from build123d import *

# Parameters (mm, degrees)
BOSS_EXTRUDE1_DEPTH      = 21.59
BOSS_EXTRUDE1_DEPTH_BACK = 21.59
SKETCH1_R                = 5.715
SKETCH3_W                = 43.18
SKETCH3_H                = 11.43
BOSS_EXTRUDE3_DEPTH      = 12.7
SKETCH4_W                = 36.83
SKETCH4_H                = 15.24
BOSS_EXTRUDE4_DEPTH      = 24.13
SKETCH7_W                = 36.83
SKETCH7_H                = 12.7
BOSS_EXTRUDE5_DEPTH      = 10.795
SKETCH5_R                = 3.175
CUT_EXTRUDE1_DEPTH       = 52.230767367
CUT_EXTRUDE5_DEPTH       = 52.230767367
FILLET1_R                = 2.54
CUT_EXTRUDE6_DEPTH       = 6.35
CUT_EXTRUDE6_DEPTH_BACK  = 6.35
SKETCH10_W               = 22.86
SKETCH10_H               = 25.4
SKETCH11_R               = 1.778
CUT_EXTRUDE7_DEPTH       = 36.017241825
SKETCH24_W               = 48.26
SKETCH24_H               = 24.13
BOSS_EXTRUDE6_DEPTH      = 2.54
SKETCH17_W               = 12.7
SKETCH17_H               = 3.175
CUT_EXTRUDE9_DEPTH       = 8.89
SKETCH18_W               = 9.525
SKETCH18_H               = 6.927192993
CUT_EXTRUDE13_DEPTH      = 45.508925283
CHAMFER1_SIZE            = 1.27
FILLET2_R                = 1.27


with BuildPart() as part:
    # Sketch1 → Boss-Extrude1 (new, two sides: drawn at the far end of the back side and taken through both)
    with BuildSketch(Plane(origin=(0, 0, 0), x_dir=(0, 0, -1), z_dir=(1, 0, 0)).offset(-BOSS_EXTRUDE1_DEPTH_BACK)):
        Circle(SKETCH1_R)
    extrude(amount=BOSS_EXTRUDE1_DEPTH + BOSS_EXTRUDE1_DEPTH_BACK)

    # Sketch3 → Boss-Extrude3 (add)
    with BuildSketch(Plane(origin=(0, 0, 0), x_dir=(1, 0, 0), z_dir=(0, 1, 0))):
        Rectangle(SKETCH3_W, SKETCH3_H)
    extrude(amount=BOSS_EXTRUDE3_DEPTH)


with BuildPart() as body_2:
    # Sketch4 → Boss-Extrude4 (new body)
    with BuildSketch(Plane.XY):
        with Locations((0, 5.08)):
            Rectangle(SKETCH4_W, SKETCH4_H)
    extrude(amount=BOSS_EXTRUDE4_DEPTH)


with BuildPart() as body_3:
    # Sketch7 → Boss-Extrude5 (new body)
    with BuildSketch(Plane.XZ.offset(2.54)):
        with Locations((0, 17.78)):
            Rectangle(SKETCH7_W, SKETCH7_H)
    extrude(amount=BOSS_EXTRUDE5_DEPTH)


with BuildPart() as cut_extrude1_tool:
    # Sketch5 → Cut-Extrude1 (new, through all)
    with BuildSketch(Plane.ZY.offset(21.59)):
        Circle(SKETCH5_R)
    extrude(amount=-CUT_EXTRUDE1_DEPTH)


with BuildPart() as part_1:
    add(part.part)

    # Cut-Extrude1: cut by cut_extrude1_tool
    add(cut_extrude1_tool.part, mode=Mode.SUBTRACT)


with BuildPart() as body_2_1:
    add(body_2.part)

    # Cut-Extrude1: cut by cut_extrude1_tool
    add(cut_extrude1_tool.part, mode=Mode.SUBTRACT)


with BuildPart() as cut_extrude5_tool:
    # Sketch6 → Cut-Extrude5 (new, through all)
    with BuildSketch(Plane(origin=(21.59, 0, 0), x_dir=(0, 0, -1), z_dir=(1, 0, 0))):
        with BuildLine():
            ThreePointArc((-19.445417037, -14.2875), (-24.13, 0), (-19.445417037, 14.2875))
            Line((-19.445417037, 14.2875), (-27.94, 14.2875))
            Line((-27.94, 14.2875), (-27.94, -14.2875))
            Line((-27.94, -14.2875), (-19.445417037, -14.2875))
        make_face()
    extrude(amount=-CUT_EXTRUDE5_DEPTH)


with BuildPart() as body_2_2:
    add(body_2_1.part)

    # Cut-Extrude5: cut by cut_extrude5_tool
    add(cut_extrude5_tool.part, mode=Mode.SUBTRACT)


with BuildPart() as body_3_1:
    add(body_3.part)

    # Cut-Extrude5: cut by cut_extrude5_tool
    add(cut_extrude5_tool.part, mode=Mode.SUBTRACT)

    # Fillet1
    fillet1_edges = [body_3_1.edges().sort_by_distance(p)[0] for p in [
        (0, -13.335, 20.11056128),
        (0, -13.335, 11.43),
    ]]
    fillet(fillet1_edges, radius=FILLET1_R)


with BuildPart() as cut_extrude6_tool:
    # Sketch10 → Cut-Extrude6 (new, two sides: drawn at the far end of the back side and taken through both)
    with BuildSketch(Plane(origin=(0, 0, 0), x_dir=(0, 0, -1), z_dir=(1, 0, 0)).offset(-CUT_EXTRUDE6_DEPTH_BACK)):
        with Locations((-8.255, -7.62)):
            Rectangle(SKETCH10_W, SKETCH10_H)
    extrude(amount=CUT_EXTRUDE6_DEPTH + CUT_EXTRUDE6_DEPTH_BACK)


with BuildPart() as part_2:
    add(part_1.part)

    # Cut-Extrude6: cut by cut_extrude6_tool
    add(cut_extrude6_tool.part, mode=Mode.SUBTRACT)


with BuildPart() as body_2_3:
    add(body_2_2.part)

    # Cut-Extrude6: cut by cut_extrude6_tool
    add(cut_extrude6_tool.part, mode=Mode.SUBTRACT)

    # Sketch11 → Cut-Extrude7 (cut, through all)
    with BuildSketch(Plane(origin=(0, 0, 0), x_dir=(0, 0, -1), z_dir=(1, 0, 0))):
        with Locations((-14.2875, 0)):
            Circle(SKETCH11_R)
    extrude(amount=-CUT_EXTRUDE7_DEPTH, mode=Mode.SUBTRACT)


with BuildPart() as body_3_2:
    add(body_3_1.part)

    # Cut-Extrude6: cut by cut_extrude6_tool
    add(cut_extrude6_tool.part, mode=Mode.SUBTRACT)


with BuildPart() as body_2_4:
    add(body_2_3.part)

    # Combine1: union body 3, part
    add(body_3_2.part)
    add(part_2.part)

    # Sketch24 → Boss-Extrude6 (add)
    with BuildSketch(Plane(origin=(0, 12.7, 0), x_dir=(1, 0, 0), z_dir=(0, 1, 0))):
        with Locations((0, -6.35)):
            Rectangle(SKETCH24_W, SKETCH24_H)
    extrude(amount=BOSS_EXTRUDE6_DEPTH)

    # Sketch17 → Cut-Extrude9 (cut)
    with BuildSketch(Plane(origin=(0, -10.005646771, -1.764265485), x_dir=(-1, 0, 0), z_dir=(0, 0.984807753012208, 0.17364817766693072))):
        with BuildLine():
            Line((-6.35, 21.666839892), (6.35, 21.666839892))
            ThreePointArc((6.35, 21.666839892), (0, 23.193431999), (-6.35, 21.666839892))
        make_face()
        with Locations((0, 20.079339892)):
            Rectangle(SKETCH17_W, SKETCH17_H)
    extrude(amount=CUT_EXTRUDE9_DEPTH, mode=Mode.SUBTRACT)

    # Sketch18 → Cut-Extrude13 (cut, through all)
    with BuildSketch(Plane(origin=(0, -13.335, 0), x_dir=(1, 0, 0), z_dir=(0, 1, 0))):
        with Locations((12.3825, -16.163596497)):
            Rectangle(SKETCH18_W, SKETCH18_H)
    extrude(amount=CUT_EXTRUDE13_DEPTH, mode=Mode.SUBTRACT)

    # Chamfer1
    chamfer1_edges = [body_2_4.edges().sort_by_distance(p)[0] for p in [
        (24.13, 15.24, 6.35),
        (24.13, 12.7, 6.35),
        (-24.13, 15.24, 6.35),
        (-24.13, 12.7, 6.35),
    ]]
    chamfer(chamfer1_edges, length=CHAMFER1_SIZE - 0.0001)  # a hair under: the kernel refuses the full size

    # Fillet2
    fillet2_edges = [body_2_4.edges().sort_by_distance(p)[0] for p in [
        (0, 12.7, 20.517477915),
    ]]
    fillet(fillet2_edges, radius=FILLET2_R)


solid = body_2_4.part
The listing builds one solid part. Answer for the finished solid, in the listing's coordinates (mm). A direction names the side the tool comes from. Give positions to 0.01 mm unless a question says otherwise; leave off trailing zeros. Write each loop counter-clockwise with the first axis right and the second up, starting at its lowest first coordinate (ties: lowest second). Pieces come first, ordered by that corner, then holes.
1) Section D-D (y = 4) is taken. Write down the section's boundary in (x, z) (3 decimals).
2) Find the intervals of material crossed by L1, parallel to Z at x = 14, y = 0 (3 decimals); L2, parallel to X at y = -10.5, z = 18.5 (3 decimals), in increasing order.
3) For a pull along X with two mould halves and no side action, classify faces 1 (the face through (18.415, 0, 14)), 2 (the face through (0, 0, -3.175)), 3 (the face through (21, 12.7, 9)), 4 (the face through (-21.59, 5, 0)) as pulls with the +X half, pulls with the -X half, needs draft (parallel to the pull), parting line crosses it, or undercut.
4) Section B-B (z = 0) is taken. Count the separate pieces of the cut face and the enclosed holes in it, and give its area (3 significant figures).
5) Section A-A (x = 16) is taken. Write down the section's boundary in (y, z) (3 decimals), and give its area (3 significant figures).
6) A tool of negligible diameter and unlimited length cuts with its end or side. For faces 5 (the face through (-18.415, 3, 14)), 6 (the face through (-8, 14, 18.415)), 7 (the face through (12, -2.54, 8)), from which of +Z, -Z, +X, -X, +Y, -Y can it reach the whole face along a straight path? Write none if from no direction.
7) Given P1, Ø5, axis at y = 5.5, z = -2.5, coming from the -X side; P2, Ø2, axis at y = -3, z = 17.5, coming from the -X side (3 decimals); P3, Ø10, axis at x = -14.5, y = -3.5, coming from the +Z side; P4, Ø5.5, axis at y = 0, z = 0, coming from the +X side, each flat-ended and moving along its own axis, determine where each tip first touches the part or whether it passes through.
Response:
1. outline: (-21.59, -5.715) - (21.59, -5.715) - (21.59, 5.715) - (18.415, 5.715) - (18.415, 23.796) - (-18.415, 23.796) - (-18.415, 5.715) - (-21.59, 5.715) - close; hole (-6.35, -3.175) - (6.35, -3.175) - (6.35, 19.685) - (-6.35, 19.685) - close; hole (7.62, 12.7) - (17.145, 12.7) - (17.145, 19.627) - (7.62, 19.627) - close
2. L1: z = -5.715 to -3.175, 3.175 to 12.7, 19.627 to 24.13
2. L2: x = -18.415 to -6.35, 6.35 to 7.62, 17.145 to 18.415
3. face 1: pulls with the +X half
3. face 2: undercut
3. face 3: needs draft
3. face 4: pulls with the -X half
4. separate pieces: 3
4. enclosed holes: 0
4. area: 584 mm2
5. outline: (-13.159, 19.627) - (12.7, 19.627) - (12.7, 19.797) arc R1.27 ccw to (12.065, 20.897) arc R24.13 ccw to (-12.065, 20.897) arc R2.54 ccw to start; (-12.995, 12.7) arc R2.54 ccw to (-10.795, 11.43) - (-2.54, 11.43) - (-2.54, 5.12) arc R5.715 ccw to (0, -5.715) - (15.24, -5.715) - (15.24, 12.7) - close; hole circle Ø6.35 at (0, 0)
5. area: 416 mm2
6. face 5: +Z, -X, -Y
6. face 6: +Z, +X, -X, +Y
6. face 7: +X, -X, -Y
7. P1: stops at x = -21.59
7. P2: stops at x = -18.415
7. P3: stops at z = 24.13
7. P4: passes through
